Autodesk Inventor part; units mm, degrees
ref_plane "YZ Plane" through (0, 0, 0) normal (1, 0, 0) x (0, 1, 0)
ref_plane "XZ Plane" through (0, 0, 0) normal (0, 1, 0) x (-1, 0, 0)
ref_plane "XY Plane" through (0, 0, 0) normal (0, 0, 1) x (1, 0, 0)
sketch "Эскиз1" plane through (0, 0, 0) normal (0, 1, 0) x (-1, 0, 0)
  circle A0 centre (0, 0) radius 10.5
  circle A1 centre (0, 0) radius 4
  line L0 (0, -3) -> (0, 3) construction
  line L1 (1.8028, -3) -> (-1.8028, -3)
  line L2 (-1.8028, 3) -> (1.8028, 3)
  circle A2 centre (0, 5.5) radius 1.25
  circle A3 centre (9.5, 0) radius 1
  circle A4 centre (-9.5, 0) radius 1
  line L3 (5.5, -6) -> (-5.5, -6)
  line L4 (-5.5, -6) -> (-5.5, 6)
  line L5 (5.5, 6) -> (5.5, -6)
  line L6 (5.5, -6) -> (-5.5, 6) construction
  line L7 (0, 10.5) -> (0, -10.5) construction
  arc A5 (1.8028, -3) -> (1.8028, 3) centre (0, 0) ccw
  arc A6 (-1.8028, 3) -> (-1.8028, -3) centre (0, 0) ccw
  arc A7 (1.8028, -3) -> (1.8028, 3) centre (0, 0) ccw
  arc A8 (-1.8028, 3) -> (-1.8028, -3) centre (0, 0) ccw
  line L8 (-5.5, 6) -> (-1.1456, 6)
  line L9 (1.1456, 6) -> (5.5, 6)
  line L10 (5.5, 6) -> (-5.5, 6)
  line L11 (-5.5, 6) -> (-5.5, 7)
  line L12 (-5.5, 7) -> (5.5, 7)
  line L13 (5.5, 7) -> (5.5, 6)
  dimension "d0" = 21
  dimension "d1" = 8
  dimension "d3" = 6
  dimension "d4" = 2.5
  dimension "d5" = 2.5
  dimension "d6" = 2
  dimension "d7" = 2
  dimension "d8" = 11
  dimension "d9" = 12
  dimension "d18" = 1
extrude "Выдавливание1" add sketch "Эскиз1" along normal blind 1 contours A4 | A0 | A3 | A1 | A2 L9 L5 L3 L4 L8 | A2 L8 L11 L12 L13 L9
extrude "Выдавливание2" add sketch "Эскиз1" along normal blind 1 from surface at 1 contours A4 | A0 | A3 | A2 L8 L11 L12 L13 L9
extrude "Выдавливание3" add sketch "Эскиз1" against normal blind 2 contours A1
extrude "Выдавливание4" add sketch "Эскиз1" against normal blind 2 contours A4 | A3
extrude "Выдавливание5" cut sketch "Эскиз1" against normal up to surface (1 mm away) from surface at 2 contours A2 L8 L11 L12 L13 L9
properties part number "Switch1"
The listing builds one solid part. Answer for the finished solid, in the listing's coordinates (mm). A direction names the side the tool comes from. Give positions to 0.01 mm unless a question says otherwise; leave off trailing zeros. Loops run counter-clockwise (first coordinate to the right, second up) from the corner with the lowest first, then second, coordinate; pieces in that order, holes last.
Item 1: A cutting plane is placed at D-D (z = -1.25). Give the vertices of the cut face in (x, y).
Derived:
outline: (-10.43, 0) - (-3.8, 0) - (-3.8, -2) - (-3.27, -2) - (-3.27, 1) - (-5.5, 1) - (-5.5, 2) - (-10.43, 2) - close; (3.27, -2) - (3.8, -2) - (3.8, 0) - (10.43, 0) - (10.43, 2) - (5.5, 2) - (5.5, 1) - (3.27, 1) - close
Item 2: A cutting plane is placed at C-C (z = 2.75). Give the vertices of the cut face in (x, y), then the cut area to 3 significant figures.
Derived:
outline: (-10.13, 0) - (-2.9, 0) - (-2.9, -2) - (-2.17, -2) - (-2.17, 1) - (-5.5, 1) - (-5.5, 2) - (-10.13, 2) - close; (2.17, -2) - (2.9, -2) - (2.9, 0) - (10.13, 0) - (10.13, 2) - (5.5, 2) - (5.5, 1) - (2.17, 1) - close
area: 28.2 mm2
Item 3: Each of these flat-tipped pins is pushed along its axis until it touches: pin 1 Ø0.8 at (y, z) = (1.5, 3) entering from +X; pin 2 Ø1 at (y, z) = (0, 1.5) entering from +X; pin 3 Ø1.5 at (y, z) = (-0.5, 6.5) entering from +X. Where does it stop, or does it pass through?
Derived:
pin 1: stops at x = 10.17
pin 2: stops at x = 10.45
pin 3: stops at x = 8.66
Item 4: A cutting plane is placed at B-B (y = -0.6). Give the vertices of the cut face in (x, z), then the cut area to 3 significant figures.
Derived:
outline: circle Ø2 at (-9.5, 0); circle Ø8 at (0, 0); circle Ø2 at (9.5, 0); hole (-1.8, -3) - (1.8, -3) arc R3.5 ccw to (1.8, 3) - (-1.8, 3) arc R3.5 ccw to start
area: 20.5 mm2
Item 5: A tool of negligible diameter and unlimited length cuts with its end or side. For faces 4 (the flat face through (0.1, 1.5, 7)), 5 (the cylindrical face through (10.3, -1, -0.6)), 6 (the flat face through (0, 0, 3)), from which of +Z, -Z, +X, -X, +Y, -Y can it reach the whole face along a straight path? Write none if from no direction.
Derived:
face 4: +Y
face 5: -Y
face 6: +Y, -Y
Item 6: Find the intervals of material crossed by line 1 along Z through (x, y) = (0, 0.7); line 2 along Y through (x, z) = (4.75, 5.5); line 3 along Y through (x, z) = (1, 8.25), in increasing order.
Derived:
line 1: z = -10.5 to -3, 3 to 4.25, 6.75 to 10.5
line 2: y = 0 to 1
line 3: y = 0 to 2
Item 7: A cutting plane is placed at A-A (x = 0). Give the vertices of the cut face in (y, z), then the cut area to 3 significant figures.
Derived:
outline: (-2, -4) - (0, -4) - (0, -10.5) - (2, -10.5) - (2, -6) - (1, -6) - (1, -3) - (-2, -3) - close; (-2, 3) - (1, 3) - (1, 4.25) - (0, 4.25) - (0, 4) - (-2, 4) - close; (0, 6.75) - (1, 6.75) - (1, 7) - (2, 7) - (2, 10.5) - (0, 10.5) - close
area: 24.5 mm2
Item 8: Determine the mould class of faces 1 (the flat face through (-9, -2, 0)), 2 (the cylindrical face through (-3.5, -0.5, -0.1)), 3 (the cylindrical face through (-10, 1, -3.2)) for opening direction X: +X half, -X half, draft (parallel to the pull), parting line (faces both ways), or undercut.
Derived:
face 1: draft
face 2: undercut
face 3: parting line
